For this review, take the finished solid that the model builds, in its own axes (mm). Face numbers are marked on the shaded views. A direction names the side the tool comes from. Round coordinates to 2 decimals unless told otherwise and drop trailing zeros. Write each loop counter-clockwise with the first axis right and the second up, starting at its lowest first coordinate (ties: lowest second). Pieces come first, ordered by that corner, then holes.
Autodesk Inventor part; units mm, degrees
ref_plane "Work Plane1" through (-35.5422, 10.3188, 19.05) normal (0, 0, 1) x (1, 0, 0)
ref_plane "YZ Plane" through (0, 0, 0) normal (1, 0, 0) x (0, 1, 0)
ref_plane "XZ Plane" through (0, 0, 0) normal (0, 1, 0) x (-1, 0, 0)
sketch "Sketch1" plane through (0, 0, 0) normal (0, 1, 0) x (-1, 0, 0)
  line L0 (-35.5422, 25.4) -> (35.5422, 25.4)
  line L1 (35.5422, -25.4) -> (-10.1422, -25.4)
  line L2 (-35.5422, 8.7376) -> (-35.5422, 25.4)
  line L3 (-10.1422, -25.4) -> (-10.1422, -2.8194)
  arc A0 (-10.1422, -2.8194) -> (-35.5422, 8.7376) centre (-33.3502, -20.1353) ccw
  line L4 (35.5422, 25.4) -> (35.5422, -25.4) construction
  line L5 (35.5422, 0) -> (41.7398, 0) construction
  arc A1 (35.5422, -25.4) -> (35.5422, 25.4) centre (-13.4082, 0) ccw
  point P0 (0, 0)
  dimension "d2" = 22.5806
  dimension "d3" = 28.956
  dimension "d4" = 16.6624
  dimension "d5" = 50.8
  dimension "d7" = 71.0844
  dimension "d8" = 45.6844
  dimension "d12" = 6.1976
extrude "Extrusion1" add sketch "Sketch1" along normal mid plane 20.6375
fillet "Fillet1" radius 6.35 2 edges at (10.1422, 0, -25.4) (10.1422, 0, -2.8194)
sketch "Sketch2" plane through (0, 10.3188, 0) normal (0, 1, 0) x (1, 0, 0)
  point P0 (0, 0)
sketch "Sketch3" plane through (0, 10.3188, 0) normal (0, 1, 0) x (1, 0, 0)
  line L0 (-36.6954, 6.35) -> (-2.5578, 6.35)
  line L1 (-2.5578, 6.35) -> (-2.5578, -12.7)
  line L2 (-2.5578, -12.7) -> (-36.6954, -12.7)
  line L3 (-36.6954, -12.7) -> (-36.6954, 6.35)
  line L4 (3.7922, 25.4) -> (-35.5422, 25.4)
  line L5 (35.5422, -25.4) -> (35.5422, -8.7376)
  point P0 (0, 0)
  dimension "d13" = 34.1376
  dimension "d14" = 19.05
  dimension "d15" = 19.05
  dimension "d16" = 38.1
extrude "Extrusion2" cut sketch "Sketch3" against normal through all
sketch "Sketch4" plane through (-35.5422, 10.3188, 25.4) normal (0, 0, 1) x (1, 0, 0)
  line L0 (4.0132, -3.9751) -> (34.1884, -3.9751)
  line L1 (34.1884, -3.9751) -> (34.1884, -16.6751)
  line L2 (34.1884, -16.6751) -> (4.0132, -16.6751)
  line L3 (4.0132, -16.6751) -> (4.0132, -3.9751)
  line L4 (71.0844, -20.6375) -> (0, -20.6375)
  line L5 (0, 0) -> (0, -20.6375)
  line L6 (38.1508, -3.9624) -> (67.1322, -3.9624)
  line L7 (67.1322, -3.9624) -> (67.1322, -16.6624)
  line L8 (67.1322, -16.6624) -> (38.1508, -16.6624)
  line L9 (38.1508, -16.6624) -> (38.1508, -3.9624)
  line L10 (0, 0) -> (71.0844, 0)
  point P0 (35.5422, -10.3188)
  point P1 (34.1884, -10.3251)
  dimension "d19" = 30.1752
  dimension "d20" = 3.9624
  dimension "d21" = 12.7
  dimension "d22" = 4.0132
  dimension "d23" = 3.9624
  dimension "d24" = 28.9814
  dimension "d25" = 3.9624
  dimension "d26" = 12.7
extrude "Extrusion3" cut sketch "Sketch4" against normal through all
sketch "Sketch5" plane through (-35.5422, -10.3188, -25.4) normal (0, 0, -1) x (-1, 0, 0)
  line L0 (-38.1508, 16.6751) -> (-34.1884, 16.6751)
  line L1 (-34.1884, 16.6751) -> (-34.1884, 3.9624)
  line L2 (-34.1884, 3.9624) -> (-38.1508, 3.9624)
  line L3 (-38.1508, 3.9624) -> (-38.1508, 16.6751)
  point P0 (-35.5422, 10.3188)
ref_plane "Work Plane1" through (-35.5422, 10.3188, 19.05) normal (0, 0, 1) x (1, 0, 0)
extrude "Extrusion4" cut sketch "Sketch5" against normal up to surface (44.45 mm away)
sketch "Sketch6" plane through (0, 10.3188, 0) normal (0, 1, 0) x (1, 0, 0)
  arc A0 (10.1422, 19.05) -> (3.7922, 25.4) centre (3.7922, 19.05) ccw
  point P0 (0, 0)
hole "Hole1" at (3.7922, 10.3188, -19.05) direction (0, -1, 0) diameter 4.7625 end through all
sketch "Sketch7" plane through (0, 10.3188, 0) normal (0, 1, 0) x (1, 0, 0)
  arc A0 (10.1422, 19.05) -> (3.7922, 25.4) centre (3.7922, 19.05) ccw construction
  line L0 (3.7922, 19.05) -> (3.7922, 25.4) construction
  point P0 (0, 0)
  dimension "d39" = 6.35
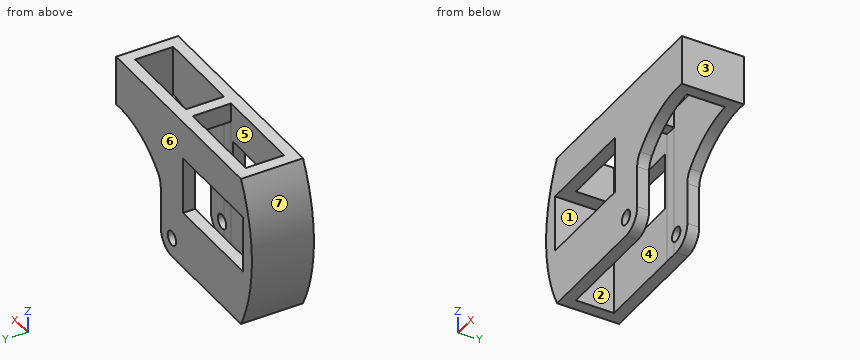
(1) For pin 1 Ø10 at (y, z) = (0, -14.5) entering from +X; pin 2 Ø2 at (x, y) = (0, -2) entering from -Z; pin 3 Ø3 at (y, z) = (-0.5, 21.5) entering from -X; pin 4 Ø3 at (x, y) = (15.5, 3.5) entering from -Z, all flat-tipped, find the tip position at first contact; note any pin that passes through.
Geometry check:
pin 1: stops at x = -31.53
pin 2: stops at z = 19.05
pin 3: stops at x = -37.99
pin 4: passes through
(2) Mouldability with a two-part tool opening along Y and no side actions: class the marked faces 5, 6 and 7 as pulls with the +Y half, pulls with the -Y half, needs draft (parallel to the pull), parting line crosses it, or undercut.
Geometry check:
face 5: undercut
face 6: pulls with the +Y half
face 7: needs draft
(3) For line 1 along Y through (x, z) = (5, 16); line 2 along Z through (x, y) = (-18, -6.5); line 3 along Y through (x, z) = (-26, -14), list the stretches that pass through material, from the lowest coordinate up.
Geometry check:
line 1: y = -10.32 to -6.34, 6.36 to 10.32
line 2: z = -25.4 to -6.35, 12.7 to 25.4
line 3: y = -10.32 to -6.36, 6.34 to 10.32
(4) We need section A-A, the plane y = 4. Give the boundary of the cut face in (x, z), and give its area (3 significant figures).
Geometry check:
outline: (-36.7, -6.35) - (-36.7, 12.7) - (-31.53, 12.7) - (-31.53, 25.4) - (-35.54, 25.4) arc R55.15 ccw to (-35.54, -25.4) - (-31.53, -25.4) - (-31.53, -6.35) - close; (-1.35, 19.05) - (2.61, 19.05) - (2.61, 25.4) - (-1.35, 25.4) - close; (31.59, 8.77) arc R28.96 cw to (35.54, 8.74) - (35.54, 25.4) - (31.59, 25.4) - close
area: 409 mm2
(5) We need section C-C, the plane z = 3. State how many separate pieces and enclosed holes the cut face has, and give its area (3 significant figures).
Geometry check:
separate pieces: 3
enclosed holes: 0
area: 249 mm2
(6) For the marked faces 1, 2, 3 and 4, list the 3-axis set-ups (+Z, -Z, +X, -X, +Y, -Y) from which the entire face can be reached by the end or side of a thin tool; tool diameter is ignored.
Geometry check:
face 1: +Y, -Y
face 2: +Z, -Z, +X
face 3: +Z, -Z, +X, +Y, -Y
face 4: +Z, -Z
(7) We need section B-B, the plane x = -11. Give the boundary of the cut face in (y, z).
Geometry check:
outline: (-10.32, -25.4) - (-6.36, -25.4) - (-6.36, -6.35) - (-10.32, -6.35) - close; (-10.32, 12.7) - (-6.36, 12.7) - (-6.36, 25.4) - (-10.32, 25.4) - close; (6.34, -25.4) - (10.32, -25.4) - (10.32, -6.35) - (6.34, -6.35) - close; (6.34, 12.7) - (10.32, 12.7) - (10.32, 25.4) - (6.34, 25.4) - close
